from build123d import *

# Parameters (mm, degrees)
SKETCH1_R           = 97.5
BOSS_EXTRUDE1_DEPTH = 5
SKETCH2_R           = 27.5
CUT_EXTRUDE1_DEPTH  = 138.976447265
SKETCH3_R           = 6.325847544
CUT_EXTRUDE2_DEPTH  = 4.064146
CIRPATTERN1_START   = 0.935854482
CIRPATTERN1_DEPTH   = 4.064145518


# Read off the part's stored shape, not the designer's step: CirPattern1
with BuildPart() as part:
    # Sketch1 → Boss-Extrude1 (new body)
    with BuildSketch(Plane(origin=(0, 0, 0), x_dir=(1, 0, 0), z_dir=(0, 1, 0))):
        with Locations(Location((0, 0, 0), (0, 0, 270))):
            Circle(SKETCH1_R)
    extrude(amount=BOSS_EXTRUDE1_DEPTH)

    # Sketch2 → Cut-Extrude1 (cut, through all)
    with BuildSketch(Plane(origin=(0, 0, 0), x_dir=(1, 0, 0), z_dir=(0, 1, 0))):
        with Locations(Location((0, 0, 0), (0, 0, 270))):
            Circle(SKETCH2_R)
    extrude(amount=CUT_EXTRUDE1_DEPTH, mode=Mode.SUBTRACT)

    # Sketch3 → Cut-Extrude2 (cut)
    with BuildSketch(Plane(origin=(0, 5, 0), x_dir=(1, 0, 0), z_dir=(0, 1, 0))):
        with Locations((-28.013239074, 0)):
            Circle(SKETCH3_R)
    extrude(amount=-CUT_EXTRUDE2_DEPTH, mode=Mode.SUBTRACT)

    # CirPattern1 outline → CirPattern1 (cut)
    with BuildSketch(Plane(origin=(0, 0, 0), x_dir=(1, 0, 0), z_dir=(0, 1, 0)).offset(CIRPATTERN1_START)):
        with BuildLine():
            ThreePointArc((8.020207871, 26.30449136), (13.75, 23.815698604), (18.770253816, 20.09794944))
            ThreePointArc((18.770253816, 20.09794944), (17.169543309, 29.738521354), (8.020207871, 26.30449136))
        make_face()
        with BuildLine():
            ThreePointArc((18.770253816, -20.09794944), (13.75, -23.815698604), (8.020207871, -26.30449136))
            ThreePointArc((8.020207871, -26.30449136), (17.169543309, -29.738521354), (18.770253816, -20.09794944))
        make_face()
    extrude(amount=CIRPATTERN1_DEPTH, mode=Mode.SUBTRACT)


solid = part.part
Design review of the part built by this model. Coordinates are the model's own, in mm. A direction names the side the tool comes from. Coordinates: 2 decimals unless noted, no trailing zeros. Order: outer loops, then holes, each group sorted by start corner. A loop starts at its lowest first (then second) coordinate and runs counter-clockwise, first axis right, second up.
Item 1: Take a section at C-C, the plane y = 2.3. Write out the cut boundary in (x, z).
Item 2: For line 1 (X direction, y = 2.65, z = 0); line 2 (Z direction, x = -15.5, y = 2.8); line 3 (X direction, y = 1.75, z = 29.5), list the stretches that pass through material, from the lowest coordinate up.
Item 3: The part is to be moulded in two halves that separate along Z. For faces 1 (the flat face through (-20, 0, 20)), 2 (the cylindrical face through (17.033, 2.939, 29.815)), 3 (the cylindrical face through (-86.5, 2.46, 44.99)), say which applies: pulls with the +Z half, pulls with the -Z half, needs draft (parallel to the pull), parting line crosses it, or undercut.
Item 4: Take a section at D-D, the plane x = 36.5. Write out the cut boundary in (y, z).
Item 5: Take a section at B-B, the plane z = 0. Write out the cut boundary in (x, y).
Item 6: For faces 4 (the flat face through (-20, 5, 20)), 5 (the cylindrical face through (17.3, 2.94, -29.66)), list the 3-axis set-ups (+Z, -Z, +X, -X, +Y, -Y) from which the entire face can be reached by the end or side of a thin tool; tool diameter is ignored.
Item 7: Take a section at A-A, the plane x = 0. Write out the cut boundary in (y, z), then the cut area to 3 significant figures.
Item 8: For pin 1 Ø1 at (x, y) = (-20.5, 2) entering from -Z; pin 2 Ø6 at (x, z) = (-30.5, -2) entering from +Y; pin 3 Ø1.5 at (y, z) = (2.5, 63) entering from -X, all flat-tipped, find the tip position at first contact; note any pin that passes through.
The answers:
1. outline: circle Ø195 at (0, 0); hole (-26.79, -6.21) arc R27.5 ccw to (8.02, -26.3) arc R6.33 ccw (long way) to (18.77, -20.1) arc R27.5 ccw to (18.77, 20.1) arc R6.33 ccw (long way) to (8.02, 26.3) arc R27.5 ccw to (-26.79, 6.21) arc R6.33 ccw (long way) to start
2. line 1: x = -97.5 to -34.34, 27.5 to 97.5
2. line 2: z = -96.26 to -22.72, 22.72 to 96.26
2. line 3: x = -92.93 to 10.46, 17.55 to 92.93
3. face 1: needs draft
3. face 2: undercut
3. face 3: parting line crosses it
4. outline: (0, -90.41) - (5, -90.41) - (5, 90.41) - (0, 90.41) - close
5. outline: (-97.5, 0) - (-27.5, 0) - (-27.5, 0.94) - (-34.34, 0.94) - (-34.34, 5) - (-97.5, 5) - close; (27.5, 0) - (97.5, 0) - (97.5, 5) - (27.5, 5) - close
6. face 4: +Z, -Z, +X, -X, +Y
6. face 5: +Y
7. outline: (0, -97.5) - (5, -97.5) - (5, -27.5) - (0, -27.5) - close; (0, 27.5) - (5, 27.5) - (5, 97.5) - (0, 97.5) - close
7. area: 700 mm2
8. pin 1: stops at z = -95.43
8. pin 2: stops at y = 0.94
8. pin 3: stops at x = -75.04
